Autodesk Inventor part; units mm, degrees
ref_plane "YZ Plane" through (0, 0, 0) normal (1, 0, 0) x (0, 1, 0)
ref_plane "XZ Plane" through (0, 0, 0) normal (0, 1, 0) x (-1, 0, 0)
ref_plane "XY Plane" through (0, 0, 0) normal (0, 0, 1) x (1, 0, 0)
sketch "Sketch1" plane through (0, 0, 0) normal (1, 0, 0) x (0, 1, 0)
  circle A0 centre (0, 0) radius 22
  dimension "d0" = 44
extrude "Extrusion1" add sketch "Sketch1" along normal blind 2.4
sketch "Sketch2" plane through (2.4, 0, 0) normal (1, 0, 0) x (0, 0, -1)
  line L0 (0, 0) -> (0, 17.5)
  circle A0 centre (0, 17.5) radius 2.75
  circle A1 centre (-15.1554, -8.75) radius 2.75
  circle A2 centre (15.1554, -8.75) radius 2.75
  dimension "d3" = 17.5
  dimension "d4" = 5.5
  dimension "d7" = 360
extrude "Extrusion2" cut sketch "Sketch2" against normal blind 2.4
sketch "Sketch3" plane through (2.4, 0, 0) normal (1, 0, 0) x (0, 0, -1)
  circle A0 centre (0, 0) radius 11
  dimension "d11" = 22
extrude "Extrusion3" add sketch "Sketch3" along normal blind 25.6
sketch "Sketch4" plane through (0, 0, 0) normal (-1, 0, 0) x (0, 0, 1)
  circle A0 centre (0, 0) radius 11
  circle A1 centre (0, 0) radius 3.9
  dimension "d14" = 7.8
extrude "Extrusion4" add sketch "Sketch4" along normal blind 9 contours A1
properties part number "SlipRing-022A-12"
CAD build for the part. Positions are in the model's coordinates, mm. A direction names the side the tool comes from. Coordinates: 2 decimals unless noted, no trailing zeros. Write each loop counter-clockwise with the first axis right and the second up, starting at its lowest first coordinate (ties: lowest second). Pieces come first, ordered by that corner, then holes. Notation, with made-up numbers: (-25.75, 79) -> (-12.75, 79) arc R9 cw to (-12.75, 94) -> close; hole circle Ø4 at (80.25, 37.5). An arc over 180 degrees is marked (long way). Return JSON: item names as keys, results as strings. Group by question number.
Q1. Flat gauge pins, fed straight in: pin 1 (1 mm diameter, centred on y = -13, z = 0.5, fed in from +X); pin 2 (1 mm diameter, centred on x = 23.5, z = 1, fed in from +Y); pin 3 (6 mm diameter, centred on x = -3.5, y = -14, fed in from +Z); pin 4 (2 mm diameter, centred on x = 1.5, z = 1.5, fed in from -Y). Where does each tip first touch, or does it go through?
Q2. Cut at A-A, the plane z = 0. Give the cut face in (x, y).
Q3. Cut at D-D, the plane y = 17.5. Give the cut face in (x, z).
Q4. Cut at B-B, the plane y = 0. Give the cut face in (x, z).
Q5. Cut at C-C, the plane y = -7. Give the cut face in (x, z).
Q6. Pull direction Z, two halves, no side cores. Call faces 4 (the face through (1.217, -9.803, -17.696)), 5 (the face through (1.183, -4.769, 21.477)), 6 (the face through (2.4, 5, 10)): released by +Z, released by -Z, zero draft, split by the parting line, or undercut.
Q7. Which spindle directions (+Z, -Z, +X, -X, +Y, -Y) get a long thin tool onto all of the face, cutting with end or side? Do faces 1 (the face through (-9, 0, 0)), 2 (the face through (15.02, 10.74, 2.38)), 3 (the face through (-4.44, -2.64, -2.87)). Say none if no direction does.
Q8. Drill centre lines: line 1 (X direction, y = 3.5, z = -12); line 2 (X direction, y = 4, z = 3); line 3 (Z direction, x = 11.5, y = 0.5). Where is each one in solid material? Low to high.
Returned:
{
 "1": {"pin 1": "stops at x = 2.4", "pin 2": "stops at y = 10.99", "pin 3": "passes through", "pin 4": "stops at y = -21.99"},
 "2": {"outline": "(-9, -3.9) -> (0, -3.9) -> (0, -22) -> (2.4, -22) -> (2.4, -11) -> (28, -11) -> (28, 11) -> (2.4, 11) -> (2.4, 14.75) -> (0, 14.75) -> (0, 3.9) -> (-9, 3.9) -> close; (0, 20.25) -> (2.4, 20.25) -> (2.4, 22) -> (0, 22) -> close"},
 "3": {"outline": "(0, -13.33) -> (2.4, -13.33) -> (2.4, -2.75) -> (0, -2.75) -> close; (0, 2.75) -> (2.4, 2.75) -> (2.4, 13.33) -> (0, 13.33) -> close"},
 "4": {"outline": "(-9, -3.9) -> (0, -3.9) -> (0, -22) -> (2.4, -22) -> (2.4, -11) -> (28, -11) -> (28, 11) -> (2.4, 11) -> (2.4, 22) -> (0, 22) -> (0, 3.9) -> (-9, 3.9) -> close"},
 "5": {"outline": "(0, -20.86) -> (2.4, -20.86) -> (2.4, -17.28) -> (0, -17.28) -> close; (0, -13.03) -> (2.4, -13.03) -> (2.4, -8.49) -> (28, -8.49) -> (28, 8.49) -> (2.4, 8.49) -> (2.4, 13.03) -> (0, 13.03) -> close; (0, 17.28) -> (2.4, 17.28) -> (2.4, 20.86) -> (0, 20.86) -> close"},
 "6": {"face 4": "undercut", "face 5": "split by the parting line", "face 6": "zero draft"},
 "7": {"face 1": "+Z, -Z, -X, +Y, -Y", "face 2": "+X", "face 3": "-X"},
 "8": {"line 1": "x = 0 to 2.4", "line 2": "x = 0 to 28", "line 3": "z = -10.99 to 10.99"}
}
